Source: CAD feature listing. Evaluate the final solid. Frame: model axes, mm. Round coordinates to 2 decimals unless told otherwise and drop trailing zeros. Order: outer loops, then holes, each group sorted by start corner. A loop starts at its lowest first (then second) coordinate and runs counter-clockwise, first axis right, second up. Notation, with made-up numbers: (75.5, -21) -> (132.5, -21) arc R36 ccw to (132.5, 15) -> close; hole circle Ø5 at (29, 25). An arc over 180 degrees is marked (long way). One line per item, written item: value. Start each with the question number.
1) Section C-C (x = -6.5). Return the cut outline in (y, z), and give its area (3 significant figures).
2) Pin query (flat end, axial travel): P1, Ø3, axis at y = 13, z = -15, coming from the +X side; P2, Ø2, axis at x = -16.5, z = -12.5, coming from the +Y side; P3, Ø5, axis at x = 1.5, z = 16, coming from the -Y side; P4, Ø1, axis at y = 4, z = 11, coming from the -X side. Return the tip coordinate at first contact, or that it passes through.
3) Ray query, L1, parallel to X at y = 10.5, z = 0; L2, parallel to Z at x = -1, y = 11.25; L3, parallel to Z at x = 7.5, y = 12.5. Return the intervals inside material, ascending.
4) Mould query, pull axis X, two halves, no side actions, for faces 1 (the face through (-10.74, 7.6, -2.38)), 2 (the face through (-17.4, 6.41, 9.86)), 3 (the face through (16.91, 14.4, 9.57)). Classes: pulls with the +X half, pulls with the -X half, needs draft (parallel to the pull), parting line crosses it, or undercut.
5) Section B-B (y = 9.75). Return the cut outline in (x, z), and give its area (3 significant figures).
6) Section A-A (x = 0). Return the cut outline in (y, z), and give its area (3 significant figures).
```python
from build123d import *

# Parameters (mm, degrees)
EXTRUDE_1_DEPTH     = 15
SKETCH_2_R          = 11
CUT_EXTRUDE_1_DEPTH = 35.034296428
FILLET_1_R          = 2


with BuildPart() as part:
    # 草图1 → 凸台-拉伸1 (new body)
    with BuildSketch(Plane(origin=(0, 0, 0), x_dir=(1, 0, 0), z_dir=(0, 1, 0))):
        Polygon((-11.547005384, -20), (11.547005384, -20), (23.094010768, 0), (11.547005384, 20), (-11.547005384, 20), (-23.094010768, 0), align=None)
    extrude(amount=EXTRUDE_1_DEPTH)

    # 草图2 → 切除-拉伸1 (cut, through all)
    with BuildSketch(Plane(origin=(0, 15, 0), x_dir=(1, 0, 0), z_dir=(0, 1, 0))):
        with Locations(Location((0, 0, 0), (0, 0, 270))):
            Circle(SKETCH_2_R)
    extrude(amount=-CUT_EXTRUDE_1_DEPTH, mode=Mode.SUBTRACT)

    # 圆角1
    fillet_1_edges = [part.edges().sort_by_distance(p)[0] for p in [
        (17.320508076, 15, 10),
        (17.320508076, 15, -10),
        (0, 15, -20),
        (-17.320508076, 15, -10),
        (-17.320508076, 15, 10),
        (0, 15, 20),
    ]]
    fillet(fillet_1_edges, radius=FILLET_1_R)


solid = part.part
```
Findings:
1. outline: (0, -20) -> (13, -20) arc R2 ccw to (15, -18) -> (15, -8.87) -> (0, -8.87) -> close; (0, 8.87) -> (15, 8.87) -> (15, 18) arc R2 ccw to (13, 20) -> (0, 20) -> close
1. area: 332 mm2
2. P1: x = 15.3
2. P2: y = 14.28
2. P3: y = 0
2. P4: x = -17.03
3. L1: -23.09 to -11, 11 to 23.09
3. L2: -20 to -10.95, 10.95 to 20
3. L3: -20 to -8.05, 8.05 to 20
4. face 1: undercut
4. face 2: pulls with the -X half
4. face 3: pulls with the +X half
5. outline: (-23.09, 0) -> (-11.55, -20) -> (11.55, -20) -> (23.09, 0) -> (11.55, 20) -> (-11.55, 20) -> close; hole circle Ø22 at (0, 0)
5. area: 1,010 mm2
6. outline: (0, -20) -> (13, -20) arc R2 ccw to (15, -18) -> (15, -11) -> (0, -11) -> close; (0, 11) -> (15, 11) -> (15, 18) arc R2 ccw to (13, 20) -> (0, 20) -> close
6. area: 268 mm2
